Here's how the part is built. I have some questions about the finished solid (model axes, mm). A direction names the side the tool comes from. Round coordinates to 2 decimals unless told otherwise and drop trailing zeros. Write each loop counter-clockwise with the first axis right and the second up, starting at its lowest first coordinate (ties: lowest second). Pieces come first, ordered by that corner, then holes. Notation, with made-up numbers: (-9, 41) - (48, 41) arc R21 ccw to (48, 56) - close; hole circle Ø10 at (-21, -7.5). An arc over 180 degrees is marked (long way). Use one line per item in the form item = value. Start each with the question number.
1. Will these pins go through, and if not, where does the flat tip stop? pin 1 (4 mm diameter, centred on y = -1.5, z = 39.5, fed in from +X); pin 2 (3 mm diameter, centred on y = 2.5, z = 17.5, fed in from -X); pin 3 (2 mm diameter, centred on x = -7.5, y = 11.5, fed in from +Z); pin 4 (9 mm diameter, centred on y = 0, z = -135, fed in from +X).
2. I want a section at D-D, the plane z = -15.5. List the corners of the cut face in (x, y) for me, plus the area to 3 significant figures.
3. Which directions (+Z, -Z, +X, -X, +Y, -Y) give clear straight access to the entire face, cutting with the end or side of a thin tool? Please do faces 1 (the flat face through (6.5, 3.1, -125)), 2 (the flat face through (0, 0, 160)).
4. I want a section at A-A, the plane y = 0. List the corners of the cut face in (x, z) for me, plus the area to 3 significant figures.
5. If I drill on line 1 along Z through (x, y) = (4.25, 0); line 2 along Y through (x, z) = (0, 54); line 3 along Z through (x, y) = (-8.5, 0), over which ranges is the centre line in solid material (lowest first)?
6. I want a section at C-C, the plane z = 138.5. List the corners of the cut face in (x, y) for me, plus the area to 3 significant figures.
7. I want a section at B-B, the plane z = -135. List the corners of the cut face in (x, y) for me.
```python
from build123d import *

# Parameters (mm, degrees)
F0_R          = 7
F1_DEPTH      = 125
F2_R          = 6
F3_DEPTH      = 35
F4_R          = 15
F5_DEPTH      = 20
F6_R          = 5
F7_DEPTH      = 15.001
F7_DEPTH_BACK = 25
F8_R          = 1


with BuildPart() as f1:
    # F0 (on Top) → F1 (new body, symmetric)
    with BuildSketch(Plane.XY):
        Circle(F0_R)
    extrude(amount=F1_DEPTH, both=True)

    # F2 (on face) → F3 (join)
    with BuildSketch(Plane.XY.offset(125)):
        Circle(F2_R)
    extrude(amount=F3_DEPTH)

    # F4 (on face) → F5 (join)
    with BuildSketch(Plane(origin=(0, 0, -125), x_dir=(1, 0, 0), z_dir=(0, 0, -1))):
        Circle(F4_R)
    extrude(amount=F5_DEPTH)

    # F6 (on Right) → F7 (cut, two sides)
    with BuildSketch(Plane.YZ) as f7_sk:
        with Locations((0, -135)):
            Circle(F6_R)
    extrude(amount=-F7_DEPTH, mode=Mode.SUBTRACT)
    extrude(f7_sk.sketch, amount=F7_DEPTH_BACK, mode=Mode.SUBTRACT)

    # F8
    f8_edges = [f1.edges().sort_by_distance(p)[0] for p in [
        (-15, 0, -145),
    ]]
    fillet(f8_edges, radius=F8_R)


solid = f1.part
```
Model answer:
q1.pin_1 = 7
q1.pin_2 = -6.93
q1.pin_3 = -125
q1.pin_4 = through
q2.outline = circle Ø14 at (0, 0)
q2.area = 154 mm2
q3.face_1 = +Z
q3.face_2 = +Z, +X, -X, +Y, -Y
q4.outline = (-15, -144) arc R1 ccw to (-14, -145) - (14, -145) arc R1 ccw to (15, -144) - (15, -140) - (-15, -140) - close; (-15, -130) - (15, -130) - (15, -125) - (7, -125) - (7, 125) - (6, 125) - (6, 160) - (-6, 160) - (-6, 125) - (-7, 125) - (-7, -125) - (-15, -125) - close
q4.area = 4,220 mm2
q5.line_1 = -145 to -140, -130 to 160
q5.line_2 = -7 to 7
q5.line_3 = -145 to -140, -130 to -125
q6.outline = circle Ø12 at (0, 0)
q6.area = 113 mm2
q7.outline = (-14.14, -5) arc R15 ccw to (14.14, -5) - close; (-14.14, 5) - (14.14, 5) arc R15 ccw to start
